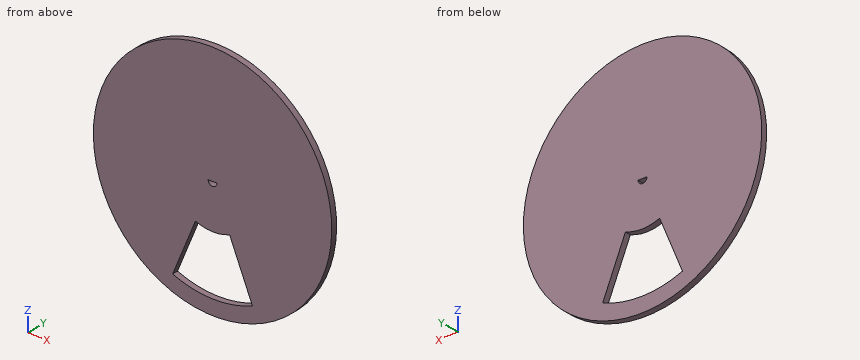
```python
from build123d import *

# Parameters (mm, degrees)
SKETCH2_R           = 40
BOSS_EXTRUDE1_DEPTH = 2
CUT_EXTRUDE1_REACH  = 58.604
CUT_EXTRUDE2_DEPTH  = 57.603886792


with BuildPart() as part:
    # Sketch2 → Boss-Extrude1 (new body)
    with BuildSketch(Plane(origin=(0, 0, 0), x_dir=(1, 0, 0), z_dir=(0, 1, 0))):
        with Locations(Location((0, 0, 0), (0, 0, 270))):
            Circle(SKETCH2_R)
    extrude(amount=BOSS_EXTRUDE1_DEPTH)

    # Sketch3 → Cut-Extrude1 (cut, up to next)
    with BuildSketch(Plane(origin=(0, 2, 0), x_dir=(1, 0, 0), z_dir=(0, 1, 0)), mode=Mode.PRIVATE) as cut_extrude1_sk1:
        with BuildLine():
            Line((-5.740251485, 13.858192988), (-13.393920133, 32.335783638))
            ThreePointArc((-13.393920133, 32.335783638), (0, 35), (13.393920133, 32.335783638))
            Line((13.393920133, 32.335783638), (5.740251485, 13.858192988))
            ThreePointArc((5.740251485, 13.858192988), (0, 15), (-5.740251485, 13.858192988))
        make_face()
    cut_extrude1_tool1 = extrude(cut_extrude1_sk1.sketch, amount=-CUT_EXTRUDE1_REACH, mode=Mode.PRIVATE) & part.part
    add(cut_extrude1_tool1.solids().sort_by_distance((0, 2, -25.661711))[0], mode=Mode.SUBTRACT)

    # Sketch5 → Cut-Extrude2 (cut, through all)
    with BuildSketch(Plane(origin=(0, 2, 0), x_dir=(1, 0, 0), z_dir=(0, 1, 0))):
        with BuildLine():
            Line((-1.5, 0), (1.5, 0))
            ThreePointArc((1.5, 0), (0, 1.5), (-1.5, 0))
        make_face()
    extrude(amount=-CUT_EXTRUDE2_DEPTH, mode=Mode.SUBTRACT)


solid = part.part
```
Input: part model. Units: mm. Frame: model coordinates. Give positions to 0.01 mm unless a question says otherwise; leave off trailing zeros. Write each loop counter-clockwise with the first axis right and the second up, starting at its lowest first coordinate (ties: lowest second). Pieces come first, ordered by that corner, then holes. Notation, with made-up numbers: (59.25, 78) - (77.25, 78) arc R29 ccw to (77.25, 115) - close; hole circle Ø6 at (87.25, 82). An arc over 180 degrees is marked (long way). Write item = value, one per line. Start each with the question number.
1) Cut plane B-B (y = 1.65). Return loops of the section in (x, z), and give its area (3 significant figures).
2) Cut plane A-A (x = 0). Return loops of the section in (y, z).
3) Pin query (flat end, axial travel): pin 1 (1 mm diameter, centred on x = -19.5, y = 1, fed in from -Z). Return the tip coordinate at first contact, or that it passes through.
4) Material intervals for L1, parallel to Z at x = 6.5, y = 0.7; L2, parallel to X at y = 0.8, z = -0.5; L3, parallel to Z at x = 10, y = 0.45, sorted ascending. Write a range as [from, to].
5) Cut plane D-D (z = 11). Return loops of the section in (x, y), and give its area (3 significant figures).
6) Cut plane C-C (x = 17). Return loops of the section in (y, z), and give its area (3 significant figures).
Answers follow:
q1.outline = circle Ø80 at (0, 0); hole (-13.39, -32.34) arc R35 ccw to (13.39, -32.34) - (5.74, -13.86) arc R15 cw to (-5.74, -13.86) - close; hole (-1.5, 0) arc R1.5 ccw to (1.5, 0) - close
q1.area = 4,630 mm^2
q2.outline = (0, -40) - (2, -40) - (2, -35) - (0, -35) - close; (0, -15) - (2, -15) - (2, -1.5) - (0, -1.5) - close; (0, 0) - (2, 0) - (2, 40) - (0, 40) - close
q3.pin_1 = -35.2
q4.L1 = [-39.47, -34.39], [-15.69, 39.47]
q4.L2 = [-40, -1.41], [1.41, 40]
q4.L3 = [-38.73, -33.54], [-24.14, 38.73]
q5.outline = (-38.46, 0) - (38.46, 0) - (38.46, 2) - (-38.46, 2) - close
q5.area = 154 mm^2
q6.outline = (0, -36.21) - (2, -36.21) - (2, 36.21) - (0, 36.21) - close
q6.area = 145 mm^2
